```python
from build123d import *

# Parameters (mm, degrees)
BOSS_EXTRUDE1_DEPTH = 116
SKETCH2_W           = 16
SKETCH2_H           = 20
BOSS_EXTRUDE2_DEPTH = 1
CUT_EXTRUDE1_DEPTH  = 163.549223314
FILLET1_R           = 2
CUT_EXTRUDE2_DEPTH  = 1
FILLET2_R           = 3
SKETCH6_R           = 2.15
CUT_EXTRUDE3_DEPTH  = 1


with BuildPart() as part:
    # Sketch1 → Boss-Extrude1 (new body)
    with BuildSketch(Plane.XY):
        with BuildLine():
            Line((-42, 18.5), (-42, -18.5))
            ThreePointArc((-42, -18.5), (-38.778174593, -26.278174593), (-31, -29.5))
            Line((-31, -29.5), (31, -29.5))
            ThreePointArc((31, -29.5), (38.778174593, -26.278174593), (42, -18.5))
            Line((42, -18.5), (42, 18.5))
            ThreePointArc((42, 18.5), (38.778174593, 26.278174593), (31, 29.5))
            Line((31, 29.5), (-31, 29.5))
            ThreePointArc((-31, 29.5), (-38.778174593, 26.278174593), (-42, 18.5))
        make_face()
        with BuildLine():
            ThreePointArc((-31, 28.5), (-38.071067812, 25.571067812), (-41, 18.5))
            Line((-41, 18.5), (-41, -18.5))
            ThreePointArc((-41, -18.5), (-38.071067812, -25.571067812), (-31, -28.5))
            Line((-31, -28.5), (31, -28.5))
            ThreePointArc((31, -28.5), (38.071067812, -25.571067812), (41, -18.5))
            Line((41, -18.5), (41, 18.5))
            ThreePointArc((41, 18.5), (38.071067812, 25.571067812), (31, 28.5))
            Line((31, 28.5), (-31, 28.5))
        make_face(mode=Mode.SUBTRACT)
    extrude(amount=-BOSS_EXTRUDE1_DEPTH)

    # Sketch2 → Boss-Extrude2 (add)
    with BuildSketch(Plane.XZ.offset(29.5)):
        with Locations((0, 10)):
            Rectangle(SKETCH2_W, SKETCH2_H)
        with Locations((0, -126)):
            Rectangle(SKETCH2_W, SKETCH2_H)
    extrude(amount=-BOSS_EXTRUDE2_DEPTH)

    # Sketch3 → Cut-Extrude1 (cut, through all)
    with BuildSketch(Plane(origin=(42, 0, 0), x_dir=(0, 0, -1), z_dir=(1, 0, 0))):
        Polygon((0, -2), (32, -2), (88, 12.5), (116, 12.5), (116, 29.5), (0, 29.5), align=None)
    extrude(amount=-CUT_EXTRUDE1_DEPTH, mode=Mode.SUBTRACT)

    # Fillet1
    fillet1_edges = [part.edges().sort_by_distance(p)[0] for p in [
        (8, -29, 20),
        (8, -29, 0),
        (-8, -29, 0),
        (-8, -29, 20),
        (-8, -29, -136),
        (-8, -29, -116),
        (8, -29, -116),
        (8, -29, -136),
        (41.5, -2, 0),
        (-41.5, 12.5, -116),
        (41.5, 12.5, -116),
        (-41.5, -2, 0),
    ]]
    fillet(fillet1_edges, radius=FILLET1_R)

    # Sketch5 → Cut-Extrude2 (cut)
    with BuildSketch(Plane.ZY.offset(42)):
        with BuildLine():
            Line((-113, -8), (-113, 12.5))
            Line((-113, 12.5), (-114, 12.5))
            ThreePointArc((-114, 12.5), (-115.414213562, 11.914213562), (-116, 10.5))
            Line((-116, 10.5), (-116, -8))
            Line((-116, -8), (-113, -8))
        make_face()
        Polygon((-88, 12.5), (-113, 12.5), (-113, -8), (-85.5, -8), (-85.5, 11.852678571), align=None)
    extrude(amount=-CUT_EXTRUDE2_DEPTH, mode=Mode.SUBTRACT)

    # Fillet2
    fillet2_edges = [part.edges().sort_by_distance(p)[0] for p in [
        (-41.5, 11.852678571, -85.5),
    ]]
    fillet(fillet2_edges, radius=FILLET2_R)

    # Sketch6 → Cut-Extrude3 (cut)
    with BuildSketch(Plane.XZ.offset(29.5)):
        with Locations((0, -124)):
            Circle(SKETCH6_R)
        with Locations((0, 8)):
            Circle(SKETCH6_R)
    extrude(amount=-CUT_EXTRUDE3_DEPTH, mode=Mode.SUBTRACT)


solid = part.part
```
Can you work these out from the model? Positions are in its coordinate system, mm. A direction names the side the tool comes from. Give positions to 0.01 mm unless a question says otherwise; leave off trailing zeros. Loops run counter-clockwise (first coordinate to the right, second up) from the corner with the lowest first, then second, coordinate; pieces in that order, holes last. Notation, with made-up numbers: M 28.5,60.5 L 71.5,60.5 A28 cw 71.5,95.5 Z; hole C 75.25,21.25 d1. An arc over 180 degrees is marked long. One line per item, written item: value.
(1) Which directions (+Z, -Z, +X, -X, +Y, -Y) give clear straight access to the entire face, cutting with the end or side of a thin tool? Please do faces 4 (the face through (37.99, -25.65, -57.19)), 5 (the face through (-41.49, 4.35, -56.53)), 6 (the face through (-34.4, -28.3, -116)), 7 (the face through (37, -27, 0)).
Returned:
face 4: +Z, -Z, +Y
face 5: +Z, +X, -X, +Y
face 6: -Z, -X, +Y, -Y
face 7: +Z, +X, +Y, -Y
(2) Suppose I cut it at A-A on z = 8. List the corners of the cut face in (x, y) for me.
Returned:
outline: M -8,-29.5 L -2.15,-29.5 L -2.15,-28.5 L -8,-28.5 Z; M 2.15,-29.5 L 8,-29.5 L 8,-28.5 L 2.15,-28.5 Z
(3) We'd pull the mould along Z, two halves only. Please class faces 1 (the face through (-37, -27, 0)), 2 (the face through (41.3, -18.3, -116)), 3 (the face through (-0.28, -29.01, 10.13)): released by +Z, released by -Z, zero draft, split by the parting line, or undercut.
Returned:
face 1: released by +Z
face 2: released by -Z
face 3: undercut
(4) Will these pins go through, and if not, where does the flat tip stop? pin 1 (0.5 mm diameter, centred on y = -29, z = -129, fed in from -X); pin 2 (1.5 mm diameter, centred on y = -21, z = -52, fed in from +X); pin 3 (11 mm diameter, centred on x = -32.5, y = -16.5, fed in from -Z); pin 4 (0.8 mm diameter, centred on y = -29, z = -130, fed in from +X).
Returned:
pin 1: x = -8
pin 2: x = 41.86
pin 3: through
pin 4: x = 8
(5) I need wall thicknesses on line 1 (Z direction, x = 0, y = -29.1); line 2 (X direction, y = -9, z = -21); line 3 (Y direction, x = 10, z = -29.5). Which ranges of each line are inside material? Lowest first, please.
Returned:
line 1: -136 to -126.15, -121.85 to 5.85, 10.15 to 20
line 2: -42 to -41, 41 to 42
line 3: -29.5 to -28.5
(6) Suppose I cut it at D-D on z = -99.5. List the corners of the cut face in (x, y) for me.
Returned:
outline: M -42,-18.5 A11 ccw -31,-29.5 L 31,-29.5 A11 ccw 42,-18.5 L 42,12.5 L 41,12.5 L 41,-18.5 A10 cw 31,-28.5 L -31,-28.5 A10 cw -41,-18.5 L -41,-8 L -42,-8 Z
(7) Suppose I cut it at C-C on y = 0.5. List the corners of the cut face in (x, z) for me, plus the area to 3 significant figures.
Returned:
outline: M -42,-85.5 L -41,-85.5 L -41,-41.66 L -42,-41.66 Z; M 41,-116 L 42,-116 L 42,-41.66 L 41,-41.66 Z
area: 118 mm^2
(8) Suppose I cut it at B-B on x = 0. List the corners of the cut face in (y, z) for me.
Returned:
outline: M -29.5,-136 L -28.5,-136 L -28.5,-126.15 L -29.5,-126.15 Z; M -29.5,-121.85 L -28.5,-121.85 L -28.5,5.85 L -29.5,5.85 Z; M -29.5,10.15 L -28.5,10.15 L -28.5,20 L -29.5,20 Z
